Could you check a few things on this model? Use its own coordinates, in mm. A direction names the side the tool comes from. Round coordinates to 2 decimals unless told otherwise and drop trailing zeros. Loops run counter-clockwise (first coordinate to the right, second up) from the corner with the lowest first, then second, coordinate; pieces in that order, holes last.
from build123d import *

# Parameters (mm, degrees)
SKETCH1_W           = 80
SKETCH1_H           = 63.35
BOSS_EXTRUDE1_DEPTH = 6.35
SKETCH2_W           = 13.333333333
SKETCH2_H           = 6.35
SKETCH2_W_2         = 26.666666666
CUT_EXTRUDE2_DEPTH  = 52.416224336
SKETCH3_R           = 20.25
CUT_EXTRUDE3_DEPTH  = 2.55
SKETCH4_R           = 20.25
CUT_EXTRUDE4_DEPTH  = 52.416224336
SKETCH5_R           = 2.1
CUT_EXTRUDE5_DEPTH  = 52.416224336
BOSS_EXTRUDE2_DEPTH = 6.35
SKETCH13_R          = 11.85
CUT_EXTRUDE8_DEPTH  = 10


with BuildPart() as part:
    # Sketch1 → Boss-Extrude1 (new body)
    with BuildSketch(Plane(origin=(0, 0, 0), x_dir=(1, 0, 0), z_dir=(0, 1, 0))):
        Rectangle(SKETCH1_W, SKETCH1_H)
    extrude(amount=BOSS_EXTRUDE1_DEPTH)

    # Sketch2 → Cut-Extrude2 (cut, through all)
    with BuildSketch(Plane(origin=(0, 6.35, 0), x_dir=(1, 0, 0), z_dir=(0, 1, 0))):
        with Locations((-33.333333334, -28.5)):
            Rectangle(SKETCH2_W, SKETCH2_H)
        with Locations((33.333333334, -28.5)):
            Rectangle(SKETCH2_W, SKETCH2_H)
        with Locations((0, -28.5)):
            Rectangle(SKETCH2_W_2, SKETCH2_H)
    extrude(amount=-CUT_EXTRUDE2_DEPTH, mode=Mode.SUBTRACT)

    # Sketch3 → Cut-Extrude3 (cut)
    with BuildSketch(Plane(origin=(0, 6.35, 0), x_dir=(1, 0, 0), z_dir=(0, 1, 0))):
        with Locations(Location((0, 3.175, 0), (0, 0, 270))):
            Circle(SKETCH3_R)
    extrude(amount=-CUT_EXTRUDE3_DEPTH, mode=Mode.SUBTRACT)

    # Sketch4 → Cut-Extrude4 (cut, through all)
    with BuildSketch(Plane(origin=(0, 6.35, 0), x_dir=(1, 0, 0), z_dir=(0, 1, 0))):
        with Locations(Location((0, 3.175, 0), (0, 0, 270))):
            Circle(SKETCH4_R)
    extrude(amount=-CUT_EXTRUDE4_DEPTH, mode=Mode.SUBTRACT)

    # Sketch5 → Cut-Extrude5 (cut, through all)
    with BuildSketch(Plane(origin=(0, 6.35, 0), x_dir=(1, 0, 0), z_dir=(0, 1, 0))):
        with Locations(Location((23.57, 26.745, 0), (0, 0, 270))):
            Circle(SKETCH5_R)
        with Locations(Location((-23.57, 26.745, 0), (0, 0, 270))):
            Circle(SKETCH5_R)
        with Locations(Location((-23.57, -20.395, 0), (0, 0, 270))):
            Circle(SKETCH5_R)
        with Locations(Location((23.57, -20.395, 0), (0, 0, 270))):
            Circle(SKETCH5_R)
    extrude(amount=-CUT_EXTRUDE5_DEPTH, mode=Mode.SUBTRACT)

    # Sketch12 → Boss-Extrude2 (add)
    with BuildSketch(Plane.XZ):
        with BuildLine():
            Line((40, 25.325), (40, -11.975))
            ThreePointArc((40, -11.975), (53.30769606, 6.675), (40, 25.325))
        make_face()
    extrude(amount=-BOSS_EXTRUDE2_DEPTH)

    # Sketch13 → Cut-Extrude8 (cut)
    with BuildSketch(Plane.XZ):
        with Locations(Location((33.585376282, 6.675, 0), (0, 0, 270))):
            Circle(SKETCH13_R)
    extrude(amount=-CUT_EXTRUDE8_DEPTH, mode=Mode.SUBTRACT)


solid = part.part
Item 1: If we section it at C-C, the plane z = -19: Please give me the cut outline in (x, y).
Results list:
outline: (-40, 0) - (-12.63, 0) - (-12.63, 6.35) - (-40, 6.35) - close; (12.63, 0) - (40, 0) - (40, 6.35) - (12.63, 6.35) - close
Item 2: If I drill on line 1 along Z through (x, y) = (34, 1.75) (3 decimals); line 2 along X through (y, z) = (0.75, 8.5); line 3 along X through (y, z) = (2.5, 12), over which ranges is the centre line in solid material (lowest first)?
Results list:
line 1: z = -31.675 to -5.168, 18.518 to 25.325
line 2: x = -40 to -16.55, 16.55 to 21.88, 45.29 to 53.22
line 3: x = -40 to -13.41, 13.41 to 23, 44.17 to 52.58
Item 3: Will these pins go through, and if not, where does the flat tip stop? pin 1 (3 mm diameter, centred on y = 4, z = 28, fed in from +X); pin 2 (3 mm diameter, centred on y = 4.5, z = 19.5, fed in from +X); pin 3 (3 mm diameter, centred on y = 1.5, z = 27.5, fed in from -X).
Results list:
pin 1: stops at x = 26.67
pin 2: stops at x = 49.73
pin 3: stops at x = -26.67
Item 4: We'd pull the mould along X, two halves only. Please class faces 1 (the flat face through (16, 0, 15)), 2 (the flat face through (-40, 3, -3)), 3 (the cylindrical face through (-21.49, 3.22, 20.12)): released by +X, released by -X, zero draft, split by the parting line, or undercut.
Results list:
face 1: zero draft
face 2: released by -X
face 3: undercut
Item 5: For faces 4 (the flat face through (-33, 3, 25.325)), 5 (the flat face through (26.667, 3, 29)), 6 (the flat face through (0, 3, 25.325)), which set-ups out of +Z, -Z, +X, -X, +Y, -Y let a thin tool reach every point of the face, with its end or its side?
Results list:
face 4: +Z, -X, +Y, -Y
face 5: +Z, +X, +Y, -Y
face 6: +Z, +Y, -Y
Item 6: If we section it at A-A, the plane x = 0: Please give me the cut outline in (y, z) (3 decimals).
Results list:
outline: (0, -31.675) - (6.35, -31.675) - (6.35, -23.425) - (0, -23.425) - close; (0, 17.075) - (6.35, 17.075) - (6.35, 25.325) - (0, 25.325) - close
Item 7: If we section it at D-D, the plane y = 1: Please give me the cut outline in (x, z) (3 decimals), then the cut area to 3 significant figures.
Results list:
outline: (-40, -31.675) - (40, -31.675) - (40, -11.975) arc R19.722 ccw to (40, 25.325) - (26.667, 25.325) - (26.667, 31.675) - (13.333, 31.675) - (13.333, 25.325) - (-13.333, 25.325) - (-13.333, 31.675) - (-26.667, 31.675) - (-26.667, 25.325) - (-40, 25.325) - close; hole circle Ø4.2 at (-23.57, -26.745); hole circle Ø4.2 at (-23.57, 20.395); hole circle Ø40.5 at (0, -3.175); hole circle Ø4.2 at (23.57, -26.745); hole circle Ø4.2 at (23.57, 20.395); hole circle Ø23.7 at (33.585, 6.675)
area: 3,310 mm2
Item 8: If we section it at B-B, the plane x = -23.57: Please give me the cut outline in (y, z) (3 decimals).
Results list:
outline: (0, -31.675) - (6.35, -31.675) - (6.35, -28.845) - (0, -28.845) - close; (0, -24.645) - (6.35, -24.645) - (6.35, 18.295) - (0, 18.295) - close; (0, 22.495) - (6.35, 22.495) - (6.35, 31.675) - (0, 31.675) - close
